```python
from build123d import *

# Parameters (mm, degrees)
F1_DEPTH = 110
F2_R     = 2
F3_DEPTH = 15
F4_R     = 1.8
F5_DEPTH = 13
F6_R     = 1


with BuildPart() as f1:
    # F0 (on Top) → F1 (new body)
    with BuildSketch(Plane.XY):
        with BuildLine():
            ThreePointArc((-6.9790131878, 1.9979447669), (-5.7, 0), (-6.9790131878, -1.9979447669))
            add(Edge.make_bspline(
                [(-6.9790131878, -1.9979447669), (0, -6.1313006259), (6.9790131878, -1.9979447669)],
                knots=[0.6075302167, 0.6075302167, 0.6075302167, 2.5340624369, 2.5340624369, 2.5340624369], degree=2, weights=[1, 0.570841362, 1]))
            ThreePointArc((6.9790131878, -1.9979447669), (5.7, 0), (6.9790131878, 1.9979447669))
            add(Edge.make_bspline(
                [(6.9790131878, 1.9979447669), (0, 6.1313006259), (-6.9790131878, 1.9979447669)],
                knots=[3.7491228703, 3.7491228703, 3.7491228703, 5.6756550905, 5.6756550905, 5.6756550905], degree=2, weights=[1, 0.570841362, 1]))
        make_face()
    extrude(amount=F1_DEPTH)

    # F2 (on face) → F3 (cut)
    with BuildSketch(Plane(origin=(0, 0, 0), x_dir=(1, 0, 0), z_dir=(0, 0, -1))):
        with Locations((2.8299042024, 0)):
            Circle(F2_R)
    extrude(amount=-F3_DEPTH, mode=Mode.SUBTRACT)

    # F4 (on face) → F5 (join)
    with BuildSketch(Plane(origin=(0, 0, 0), x_dir=(1, 0, 0), z_dir=(0, 0, -1))):
        with Locations((-2.8299042024, 0)):
            Circle(F4_R)
    extrude(amount=F5_DEPTH)

    # F6
    f6_edges = [f1.edges().sort_by_distance(p)[0] for p in [
        (-4.629904, 0, -13),
    ]]
    fillet(f6_edges, radius=F6_R)


solid = f1.part
```
The listing builds one solid part. Answer for the finished solid, in the listing's coordinates (mm). A direction names the side the tool comes from. Give positions to 0.01 mm unless a question says otherwise; leave off trailing zeros. One line per item, written item: value.
1. Find the intervals of material crossed by probe 1 along Z at (x, y) = (1.5, 1); probe 2 along Z at (x, y) = (0, 2); probe 3 along Y at (x, z) = (6, 52), in increasing order.
Found:
probe 1: 15 to 110
probe 2: 0 to 110
probe 3: -2.48 to -1.11, 1.11 to 2.48
2. For faces 1 (the face through (4.677, 0.766, 7.395)), 2 (the face through (0, 0, 110)), determine the directions among +Z, -Z, +X, -X, +Y, -Y from which every point of the face is accessible in a straight line to the end or side of a thin tool.
Found:
face 1: -Z
face 2: +Z, +X, -X, +Y, -Y
3. Each of these flat-tipped pins is pushed along its axis until it touches: P1, Ø1.5, axis at y = -1, z = 89, coming from the -X side; P2, Ø1.5, axis at x = 2, z = 94, coming from the +Y side; P3, Ø1.2, axis at x = 3.5, y = 1, coming from the -Z side. Where does it stop, or does it pass through?
Found:
P1: x = -6.57
P2: y = 3.46
P3: z = 15
4. For a pull along Y with two mould halves and no side action, classify faces 3 (the face through (0, 0, 0)), 4 (the face through (-1.1, -0.5, -5.9)), 5 (the face through (3, 0, 15)) as pulls with the +Y half, pulls with the -Y half, needs draft (parallel to the pull), parting line crosses it, or undercut.
Found:
face 3: needs draft
face 4: parting line crosses it
face 5: undercut
